Geometry check sheet. Reference: the model listing, model coordinates, mm. A direction names the side the tool comes from. Round coordinates to 2 decimals unless told otherwise and drop trailing zeros. Order: outer loops, then holes, each group sorted by start corner. A loop starts at its lowest first (then second) coordinate and runs counter-clockwise, first axis right, second up.
(1) Thickness scan on L1, parallel to X at y = 10, z = -4.75; L2, parallel to Z at x = 0, y = 7.5; L3, parallel to Y at x = 31, z = 1.25. Record the ranges inside material, lowest first.
(2) Set-up check for faces 1 (the face through (51, -13, -2)), 2 (the face through (-19.184, -1.349, 1.014)), 3 (the face through (50, 0, 1)): record each of +Z, -Z, +X, -X, +Y, -Y from which the full face is reachable in a straight line by a thin tool's end or side.
(3) Gauge pin test, flat ends, axial feed: P1, Ø1, axis at x = 50.5, z = -4, coming from the -Y side; P2, Ø4, axis at x = -8.5, y = 5.5, coming from the -Z side; P3, Ø2, axis at x = -51, z = -1.5, coming from the +Y side; P4, Ø2.5, axis at y = -10, z = -3, coming from the +X side. Record the tip position at first contact, or that the pin passes through.
(4) Cross-section at D-D on x = 2.5. Enter the section's corners in (y, z), and give its area (3 significant figures).
(5) Draft check along Z on faces 4 (the face through (-1, 0, 0)), 5 (the face through (-50, -14, 1)), 6 (the face through (-51.014, 9.425, -1.614)), 7 (the face through (-51.01, -11.33, -2.31)). Enter one of: pulls with the +Z half, pulls with the -Z half, needs draft (parallel to the pull), parting line crosses it, or undercut.
(6) Cross-section at C-C on y = 10. Enter the section's corners in (x, z).
(7) Cross-section at B-B on x = -33.5. Enter the section's corners in (y, z), and give its area (3 significant figures).
(8) Cross-section at A-A on z = -3. Count the separate pieces of the cut face and the enclosed holes in it, and give its area (3 significant figures).
from build123d import *

# Parameters (mm, degrees)
SKETCH1_W           = 100
SKETCH1_H           = 30
BOSS_EXTRUDE1_DEPTH = 2
SKETCH2_W           = 2
SKETCH2_H           = 6
BOSS_EXTRUDE2_DEPTH = 8
SKETCH3_R           = 1.5
CUT_EXTRUDE1_DEPTH  = 105
CUT_EXTRUDE2_REACH  = 10
SKETCH4_R           = 1.5
SKETCH4_R_2         = 4


with BuildPart() as part:
    # Sketch1 → Boss-Extrude1 (new body)
    with BuildSketch(Plane.XY):
        Rectangle(SKETCH1_W, SKETCH1_H)
    extrude(amount=BOSS_EXTRUDE1_DEPTH)

    # Sketch2 → Boss-Extrude2 (add)
    with BuildSketch(Plane.XY.offset(2)):
        with Locations((-51, 10)):
            Rectangle(SKETCH2_W, SKETCH2_H)
        with Locations((-51, -10)):
            Rectangle(SKETCH2_W, SKETCH2_H)
        with Locations((51, 10)):
            Rectangle(SKETCH2_W, SKETCH2_H)
        with Locations((51, -10)):
            Rectangle(SKETCH2_W, SKETCH2_H)
    extrude(amount=-BOSS_EXTRUDE2_DEPTH)

    # Sketch3 → Cut-Extrude1 (cut, through all)
    with BuildSketch(Plane.ZY.offset(52)):
        with Locations((-3, 10)):
            Circle(SKETCH3_R)
        with Locations((-3, -10)):
            Circle(SKETCH3_R)
    extrude(amount=-CUT_EXTRUDE1_DEPTH, mode=Mode.SUBTRACT)

    # Sketch4 → Cut-Extrude2 (cut, up to next)
    with BuildSketch(Plane.XY.offset(2), mode=Mode.PRIVATE) as cut_extrude2_sk1:
        with Locations((-40.502306205, -6.199754272)):
            Circle(SKETCH4_R)
    cut_extrude2_tool1 = extrude(cut_extrude2_sk1.sketch, amount=-CUT_EXTRUDE2_REACH, mode=Mode.PRIVATE) & part.part
    add(cut_extrude2_tool1.solids().sort_by_distance((-40.502306, -6.199754, 2))[0], mode=Mode.SUBTRACT)
    # Sketch4 → Cut-Extrude2 (cut, up to next)
    with BuildSketch(Plane.XY.offset(2), mode=Mode.PRIVATE) as cut_extrude2_sk2:
        with Locations((-15.497693795, -6.199754272)):
            Circle(SKETCH4_R)
    cut_extrude2_tool2 = extrude(cut_extrude2_sk2.sketch, amount=-CUT_EXTRUDE2_REACH, mode=Mode.PRIVATE) & part.part
    add(cut_extrude2_tool2.solids().sort_by_distance((-15.497694, -6.199754, 2))[0], mode=Mode.SUBTRACT)
    # Sketch4 → Cut-Extrude2 (cut, up to next)
    with BuildSketch(Plane.XY.offset(2), mode=Mode.PRIVATE) as cut_extrude2_sk3:
        with Locations((-8.604808795, -7.2)):
            Circle(SKETCH4_R)
    cut_extrude2_tool3 = extrude(cut_extrude2_sk3.sketch, amount=-CUT_EXTRUDE2_REACH, mode=Mode.PRIVATE) & part.part
    add(cut_extrude2_tool3.solids().sort_by_distance((-8.604809, -7.2, 2))[0], mode=Mode.SUBTRACT)
    # Sketch4 → Cut-Extrude2 (cut, up to next)
    with BuildSketch(Plane.XY.offset(2), mode=Mode.PRIVATE) as cut_extrude2_sk4:
        with Locations((16.399709937, -7.2)):
            Circle(SKETCH4_R)
    cut_extrude2_tool4 = extrude(cut_extrude2_sk4.sketch, amount=-CUT_EXTRUDE2_REACH, mode=Mode.PRIVATE) & part.part
    add(cut_extrude2_tool4.solids().sort_by_distance((16.39971, -7.2, 2))[0], mode=Mode.SUBTRACT)
    # Sketch4 → Cut-Extrude2 (cut, up to next)
    with BuildSketch(Plane.XY.offset(2), mode=Mode.PRIVATE) as cut_extrude2_sk5:
        with Locations((28.430538533, -7.2)):
            Circle(SKETCH4_R_2)
    cut_extrude2_tool5 = extrude(cut_extrude2_sk5.sketch, amount=-CUT_EXTRUDE2_REACH, mode=Mode.PRIVATE) & part.part
    add(cut_extrude2_tool5.solids().sort_by_distance((28.430539, -7.2, 2))[0], mode=Mode.SUBTRACT)
    # Sketch4 → Cut-Extrude2 (cut, up to next)
    with BuildSketch(Plane.XY.offset(2), mode=Mode.PRIVATE) as cut_extrude2_sk6:
        with BuildLine():
            Line((-35.352440505, -0.712200048), (-20.647559495, -0.712200048))
            ThreePointArc((-20.647559495, -0.712200048), (-19.168422859, -1.366037052), (-18.65640049, -2.900045237))
            Line((-18.65640049, -2.900045237), (-19.2789871, -9.499463306))
            ThreePointArc((-19.2789871, -9.499463306), (-19.92398311, -10.790754753), (-21.270146105, -11.311618117))
            Line((-21.270146105, -11.311618117), (-34.729853895, -11.311618117))
            ThreePointArc((-34.729853895, -11.311618117), (-36.07601689, -10.790754753), (-36.7210129, -9.499463306))
            Line((-36.7210129, -9.499463306), (-37.34359951, -2.900045237))
            ThreePointArc((-37.34359951, -2.900045237), (-36.831577141, -1.366037052), (-35.352440505, -0.712200048))
        make_face()
    cut_extrude2_tool6 = extrude(cut_extrude2_sk6.sketch, amount=-CUT_EXTRUDE2_REACH, mode=Mode.PRIVATE) & part.part
    add(cut_extrude2_tool6.solids().sort_by_distance((-28, -5.931102, 2))[0], mode=Mode.SUBTRACT)
    # Sketch4 → Cut-Extrude2 (cut, up to next)
    with BuildSketch(Plane.XY.offset(2), mode=Mode.PRIVATE) as cut_extrude2_sk7:
        with BuildLine():
            Line((-3.454989934, -1.718769673), (11.249891076, -1.718769673))
            ThreePointArc((11.249891076, -1.718769673), (12.729090854, -2.372676058), (13.241032451, -3.906801654))
            Line((13.241032451, -3.906801654), (12.618390941, -10.500186773))
            ThreePointArc((12.618390941, -10.500186773), (11.973343181, -11.791354569), (10.627249567, -12.312154791))
            Line((10.627249567, -12.312154791), (-2.832348424, -12.312154791))
            ThreePointArc((-2.832348424, -12.312154791), (-4.178442039, -11.791354569), (-4.823489799, -10.500186773))
            Line((-4.823489799, -10.500186773), (-5.446131309, -3.906801654))
            ThreePointArc((-5.446131309, -3.906801654), (-4.934189711, -2.372676058), (-3.454989934, -1.718769673))
        make_face()
    cut_extrude2_tool7 = extrude(cut_extrude2_sk7.sketch, amount=-CUT_EXTRUDE2_REACH, mode=Mode.PRIVATE) & part.part
    add(cut_extrude2_tool7.solids().sort_by_distance((3.897451, -6.934685, 2))[0], mode=Mode.SUBTRACT)


solid = part.part
Found:
1. L1: x = -52 to -50, 50 to 52
1. L2: z = 0 to 2
1. L3: y = -15 to -10.27, -4.13 to 15
2. face 1: +Z, -Z, +X, -Y
2. face 2: +Z, -Z
2. face 3: +Z, -Z, +X
3. P1: stops at y = -13
3. P2: stops at z = 0
3. P3: stops at y = 13
3. P4: passes through
4. outline: (-15, 0) - (-12.31, 0) - (-12.31, 2) - (-15, 2) - close; (-1.72, 0) - (15, 0) - (15, 2) - (-1.72, 2) - close
4. area: 38.8 mm2
5. face 4: pulls with the -Z half
5. face 5: needs draft
5. face 6: undercut
5. face 7: undercut
6. outline: (-52, -6) - (-50, -6) - (-50, -4.5) - (-52, -4.5) - close; (-52, -1.5) - (-50, -1.5) - (-50, 0) - (50, 0) - (50, -1.5) - (52, -1.5) - (52, 2) - (-52, 2) - close; (50, -6) - (52, -6) - (52, -4.5) - (50, -4.5) - close
7. outline: (-15, 0) - (-11.31, 0) - (-11.31, 2) - (-15, 2) - close; (-0.71, 0) - (15, 0) - (15, 2) - (-0.71, 2) - close
7. area: 38.8 mm2
8. separate pieces: 8
8. enclosed holes: 0
8. area: 24.0 mm2
